Work out the finished part from the listing and answer in its coordinate system (mm). A direction names the side the tool comes from. Coordinates: 2 decimals unless noted, no trailing zeros. Write each loop counter-clockwise with the first axis right and the second up, starting at its lowest first coordinate (ties: lowest second). Pieces come first, ordered by that corner, then holes. Notation, with made-up numbers: (21, 72) - (66, 72) arc R22 ccw to (66, 102) - close; hole circle Ø4 at (-11, -7.5). An arc over 180 degrees is marked (long way). One line per item, written item: value.
```python
from build123d import *

# Parameters (mm, degrees)
F0_W     = 57.45079
F0_H     = 16.242632
F1_DEPTH = 25.4
F2_W     = 51.598368
F2_H     = 9.389651
F3_DEPTH = 20.32
F4_W     = 8.826647
F4_H     = 3.600052
F5_DEPTH = 35.306
F7_DEPTH = 25.4


with BuildPart() as f1:
    # F0 (on Top) → F1 (new body)
    with BuildSketch(Plane.XY):
        with Locations((-0.150396, -0.30079)):
            Rectangle(F0_W, F0_H)
    extrude(amount=F1_DEPTH)

    # F2 (on face) → F3 (cut)
    with BuildSketch(Plane.XY.offset(25.4)):
        with Locations((1.131601, -0.038353)):
            Rectangle(F2_W, F2_H)
    extrude(amount=-F3_DEPTH, mode=Mode.SUBTRACT)

    # F4 (on face) → F5 (cut)
    with BuildSketch(Plane.YZ.offset(28.574999)):
        with Locations((-0.108496, 7.22357)):
            Rectangle(F4_W, F4_H)
    extrude(amount=-F5_DEPTH, mode=Mode.SUBTRACT)

    # F6 (on face) → F7 (cut)
    with BuildSketch(Plane.XZ.offset(8.422106)):
        with BuildLine():
            Line((-18.629054, 5.46905), (26.788274, 5.46905))
            Line((26.788274, 5.46905), (26.815441, 6.593401))
            Line((26.815441, 6.593401), (-18.222148, 6.593401))
            ThreePointArc((-18.222148, 6.593401), (-20.923448, 8.422133), (-22.056237, 11.48123))
            Line((-22.056237, 11.48123), (-23.254463, 11.616431))
            ThreePointArc((-23.254463, 11.616431), (-21.942804, 7.789534), (-18.629054, 5.46905))
        make_face()
    extrude(amount=-F7_DEPTH, mode=Mode.SUBTRACT)


solid = f1.part
```
Item 1: Which of the six approach directions +Z, -Z, +X, -X, +Y, -Y give full straight-line access (tool end or side, diameter ignored) to faces 1 (the face through (-20.895, -6.603, 8.386)), 2 (the face through (-24.668, 0, 15)), 3 (the face through (28.575, 0, 13)), 4 (the face through (28, -4.522, 7))?
Evaluation:
face 1: +Y, -Y
face 2: +Z
face 3: +Z, -Z, +X, +Y, -Y
face 4: +X
Item 2: Section A-A, the plane x = 24 is taken. Determine the outline of the cut face in (y, z).
Evaluation:
outline: (-8.42, 0) - (7.82, 0) - (7.82, 5.47) - (4.66, 5.47) - (4.66, 5.08) - (-4.73, 5.08) - (-4.73, 5.47) - (-8.42, 5.47) - close; (-8.42, 6.59) - (-4.73, 6.59) - (-4.73, 25.4) - (-8.42, 25.4) - close; (4.66, 6.59) - (7.82, 6.59) - (7.82, 25.4) - (4.66, 25.4) - close
Item 3: Determine the mould class of faces 5 (the face through (-28.876, 0, 13)), 6 (the face through (1, 4.656, 18)), 7 (the face through (28, 0, 5.424)) for opening direction X: +X half, -X half, draft (parallel to the pull), parting line (faces both ways), or undercut.
Evaluation:
face 5: -X half
face 6: undercut
face 7: draft
Item 4: Consider probe 1 along X at (y, z) = (-0.5, 12) (3 decimals); probe 2 along Z at (x, y) = (-3, 5); probe 3 along Y at (x, z) = (-11, 11.25). Determine where each line is inside the solid, lowest interval first.
Evaluation:
probe 1: x = -28.876 to -24.668, 26.931 to 28.575
probe 2: z = 0 to 5.47, 6.59 to 25.4
probe 3: y = -8.42 to -4.73, 4.66 to 7.82
Item 5: Section B-B, the plane y = -5.75 is taken. Determine the outline of the cut face in (x, z) (3 decimals).
Evaluation:
outline: (-28.876, 0) - (28.575, 0) - (28.575, 25.4) - (-28.876, 25.4) - close; hole (-23.254, 11.616) arc R6.532 ccw to (-18.629, 5.469) - (26.788, 5.469) - (26.815, 6.593) - (-18.222, 6.593) arc R5.338 cw to (-22.056, 11.481) - close
Item 6: Section C-C, the plane z = 10.5 is taken. Determine the outline of the cut face in (x, y) (3 decimals), then the cut area to 3 significant figures.
Evaluation:
outline: (-28.876, -8.422) - (-23.141, -8.422) - (-23.141, -4.733) - (-24.668, -4.733) - (-24.668, 4.656) - (-23.141, 4.656) - (-23.141, 7.821) - (-28.876, 7.821) - close; (-21.921, -8.422) - (28.575, -8.422) - (28.575, 7.821) - (-21.921, 7.821) - (-21.921, 4.656) - (26.931, 4.656) - (26.931, -4.733) - (-21.921, -4.733) - close
area: 440 mm2
Item 7: Section D-D, the plane y = -0.5 is taken. Determine the outline of the cut face in (x, z) (3 decimals).
Evaluation:
outline: (-28.876, 0) - (28.575, 0) - (28.575, 5.424) - (26.931, 5.424) - (26.931, 5.08) - (-24.668, 5.08) - (-24.668, 25.4) - (-28.876, 25.4) - close; (26.931, 9.024) - (28.575, 9.024) - (28.575, 25.4) - (26.931, 25.4) - close
